CAD build for the part. Positions are in the model's coordinates, mm. Face numbers are marked on the shaded views. Give positions to 0.01 mm unless a question says otherwise; leave off trailing zeros. Write each loop counter-clockwise with the first axis right and the second up, starting at its lowest first coordinate (ties: lowest second). Pieces come first, ordered by that corner, then holes. Notation, with made-up numbers: M 86,-24 L 95,-24 A10 ccw 95,-14 Z; hole C 43.25,-22.75 d10. An arc over 180 degrees is marked long. One line per question, with ' | ' between items. Start each with the question number.
1. Wall check: L1, parallel to Y at x = -2.75, z = 1.75; L2, parallel to X at y = 2.25, z = 0; L3, parallel to Y at x = -2.25, z = 2.5. Give the ranges that are in metal, low to high.
2. Cut at A-A, the plane y = 5.5. Write the cut outline in (x, z), then the cut area to 3 significant figures.
3. Flat gauge pins, fed straight in: pin 1 (2.5 mm diameter, centred on x = 0, z = 0, fed in from +Y); pin 2 (3 mm diameter, centred on x = 2, y = 6, fed in from -Z); pin 3 (3 mm diameter, centred on y = -4, z = -1.5, fed in from -X). Where does each tip first touch, or does it go through?
4. Cut at B-B, the plane y = -1.25. Write the cut outline in (x, z), then the cut area to 3 significant figures.
5. Pull direction Y, two halves, no side cores. Call the marked faces 1 and 2: released by +Y, released by -Y, zero draft, split by the parting line, or undercut.
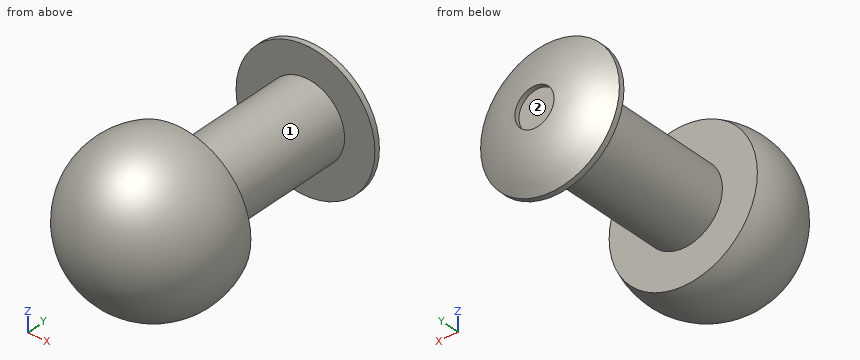
```python
from build123d import *

# Parameters (mm, degrees)
SKETCH1_R           = 2
BOSS_EXTRUDE1_DEPTH = 8
CUT_EXTRUDE1_START  = 11
SKETCH4_R           = 1
CUT_EXTRUDE1_DEPTH  = 2


with BuildPart() as part:
    # Sketch1 → Boss-Extrude1 (new body)
    with BuildSketch(Plane(origin=(0, 0, 0), x_dir=(1, 0, 0), z_dir=(0, 1, 0))):
        with Locations(Location((0, 0, 0), (0, 0, 270))):
            Circle(SKETCH1_R)
    extrude(amount=BOSS_EXTRUDE1_DEPTH)

    # Sketch2 → Revolve1 (revolve)
    with BuildSketch(Plane.XY):
        with BuildLine():
            Line((0, 0), (-3.78822299, 0))
            ThreePointArc((-3.78822299, 0), (-3.344172104, -3.752614622), (0, -5.512106206))
            Line((0, -5.512106206), (0, 0))
        make_face()
    revolve(axis=Axis((0, 0, 0), (0, -1, 0)))

    # Sketch3 → Revolve2 (revolve)
    with BuildSketch(Plane.XY):
        with BuildLine():
            ThreePointArc((-3.547394753, 8.281571529), (-1.865198603, 9.097729481), (0, 9.227851973))
            Line((0, 9.227851973), (0, 8))
            Line((0, 8), (-3.547394753, 8))
            Line((-3.547394753, 8), (-3.547394753, 8.281571529))
        make_face()
    revolve(axis=Axis((0, 8, 0), (0, 1, 0)))

    # Sketch4 → Cut-Extrude1 (cut)
    with BuildSketch(Plane(origin=(0, 0, 0), x_dir=(1, 0, 0), z_dir=(0, 1, 0)).offset(CUT_EXTRUDE1_START)):
        with Locations(Location((0, 0, 0), (0, 0, 270))):
            Circle(SKETCH4_R)
    extrude(amount=-CUT_EXTRUDE1_DEPTH, mode=Mode.SUBTRACT)


solid = part.part
```
Here are the results:
1) L1: -3.87 to 0, 8 to 8.48 | L2: -2 to 2 | L3: -3.72 to 0, 8 to 8.41
2) outline: C 0,0 d4 | area: 12.6 mm^2
3) pin 1: y = 9.25 | pin 2: z = -1.94 | pin 3: x = -3.79
4) outline: C 0,0 d8.11 | area: 51.6 mm^2
5) face 1: undercut | face 2: released by +Y
